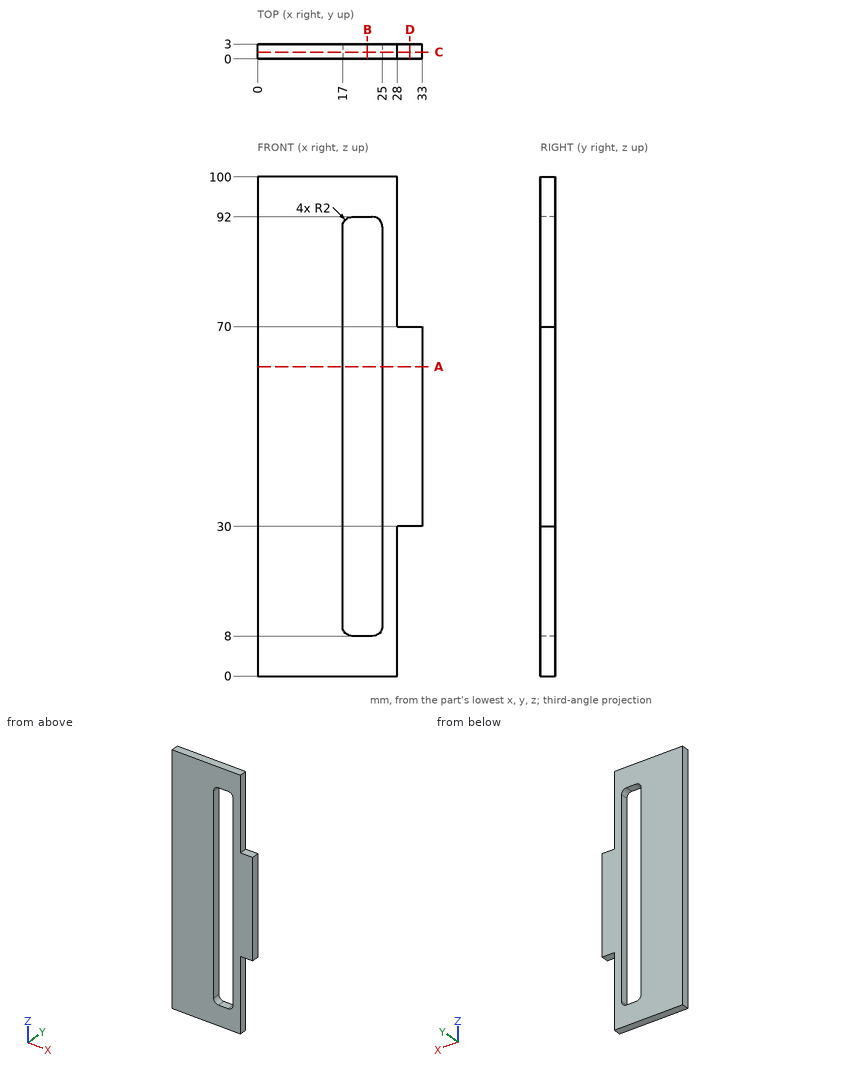
Geometry: see drawing. Coordinates: mm, zero at the bounding-box minimum. Give positions to 0.01 mm unless a question says otherwise; leave off trailing zeros. Order: outer loops, then holes, each group sorted by start corner. A loop starts at its lowest first (then second) coordinate and runs counter-clockwise, first axis right, second up. Notation, with made-up numbers: M 1.25,58 L 21.25,58 A13 cw 21.25,75 Z; hole C 39,1.25 d8. An arc over 180 degrees is marked long. Answer as a JSON object with one key per item and string values.
1. Cut plane A-A, the plane z = 62. Output: boundary loops of the cut face in (x, y).
Result sheet:
{"outline": "M 0,0 L 17,0 L 17,3 L 0,3 Z; M 25,0 L 33,0 L 33,3 L 25,3 Z"}
2. Cut plane C-C, the plane y = 1.35. Output: boundary loops of the cut face in (x, z).
Result sheet:
{"outline": "M 0,0 L 28,0 L 28,30 L 33,30 L 33,70 L 28,70 L 28,100 L 0,100 Z; hole M 17,10 A2 ccw 19,8 L 23,8 A2 ccw 25,10 L 25,90 A2 ccw 23,92 L 19,92 A2 ccw 17,90 Z"}
3. First-contact query: P1, Ø0.9, axis at y = 1.5, z = 80, coming from the +X side; P2, Ø1.5, axis at x = 30.5, y = 1.5, coming from the +Z side. Flat tips, straight axial feed; report the tip coordinate or a pass-through.
Result sheet:
{"P1": "x = 28", "P2": "z = 70"}
4. Cut plane D-D, the plane x = 30.5. Output: boundary loops of the cut face in (y, z), and give its area (3 significant figures).
Result sheet:
{"outline": "M 0,30 L 3,30 L 3,70 L 0,70 Z", "area": "120 mm²"}
5. Cut plane B-B, the plane x = 22. Output: boundary loops of the cut face in (y, z).
Result sheet:
{"outline": "M 0,0 L 3,0 L 3,8 L 0,8 Z; M 0,92 L 3,92 L 3,100 L 0,100 Z"}
6. Ray query, line 1 (X direction, y = 2.35, z = 88); line 2 (X direction, y = 0.6, z = 39); line 3 (Z direction, x = 21, y = 0.25). Return the intervals inside material, ascending. Write a range as [from, to].
Result sheet:
{"line 1": "[0, 17], [25, 28]", "line 2": "[0, 17], [25, 33]", "line 3": "[0, 8], [92, 100]"}
